Check sheet for the drawn part. Datum: minimum x, y, z corner. Units: mm. A direction names the side the tool comes from. Give positions to 0.01 mm unless a question says otherwise; leave off trailing zeros. Write each loop counter-clockwise with the first axis right and the second up, starting at its lowest first coordinate (ties: lowest second). Pieces come first, ordered by that corner, then holes. Notation, with made-up numbers: M -36,-32.75 L -7,-32.75 A22 ccw -7,1.25 Z; hole C 21.5,45 d1. An arc over 180 degrees is marked long. Write item = value, one per line. Start each with the question number.
1) Sectioned sample at A-A, the plane x = 41. Record the cut outline in (y, z).
2) Gauge pin test, flat ends, axial feed: pin 1 (1.8 mm diameter, centred on y = 2.5, z = 25, fed in from +X); pin 2 (6 mm diameter, centred on x = 5.5, z = 37, fed in from -Y); pin 3 (6.5 mm diameter, centred on y = 2, z = 35.5, fed in from -X). Record the tip position at first contact, or that the pin passes through.
3) Set-up check for the marked faces 1, 2 and 3: record each of +Z, -Z, +X, -X, +Y, -Y from which the full face is reachable in a straight line by a thin tool's end or side.
4) Scan lines: L1, parallel to Z at x = 51, y = 2.75; L2, parallel to X at y = 4.5, z = 51; L3, parallel to Y at x = 74, z = 57. Record each from-to range of solid material in increasing order.
5) Sectioned sample at B-B, the plane z = 47.5. Record the cut outline in (x, y).
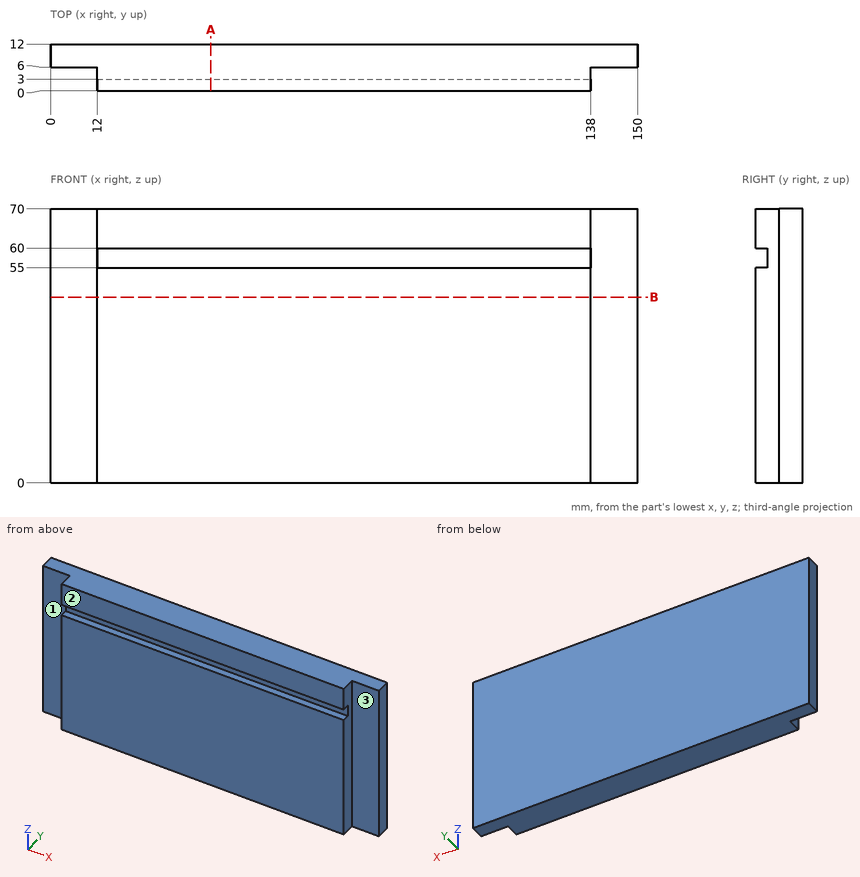
Data:
q1.outline = M 0,0 L 12,0 L 12,70 L 0,70 L 0,60 L 3,60 L 3,55 L 0,55 Z
q2.pin_1 = 138
q2.pin_2 = 6
q2.pin_3 = 12
q3.face_1 = +Z, -Z, -X, -Y
q3.face_2 = +Z, -Z, +X, -X, -Y
q3.face_3 = +Z, -Z, +X, -Y
q4.L1 = 0 to 55, 60 to 70
q4.L2 = 12 to 138
q4.L3 = 3 to 12
q5.outline = M 0,6 L 12,6 L 12,0 L 138,0 L 138,6 L 150,6 L 150,12 L 0,12 Z
